Check sheet for the modelled part. Datum: model origin and axes. Units: mm. Face numbers are marked on the shaded views. A direction names the side the tool comes from. Coordinates: 2 decimals unless noted, no trailing zeros. Order: outer loops, then holes, each group sorted by start corner. A loop starts at its lowest first (then second) coordinate and runs counter-clockwise, first axis right, second up.
1. Cross-section at A-A (y = 81.5). Enter the section's corners in (x, z).
2. Gauge pin test, flat ends, axial feed: pin 1 Ø9 at (y, z) = (16.5, 39.5) entering from +X; pin 2 Ø5 at (x, z) = (-20.5, 28) entering from +Y; pin 3 Ø1 at (y, z) = (60.5, 18) entering from +X; pin 4 Ø16 at (x, y) = (-20.5, 47) entering from -Z. Record the tip position at first contact, or that the pin passes through.
3. Set-up check for the marked faces 1, 2, 3 and 4: record each of +Z, -Z, +X, -X, +Y, -Y from which the full face is reachable in a straight line by a thin tool's end or side.
4. Draft check along X on the marked faces 5, 6 and 7. Enter one of: released by +X, released by -X, zero draft, split by the parting line, or undercut.
5. Cross-section at B-B (x = -16.5). Enter the section's corners in (y, z), then the cut area to 3 significant figures.
6. Cross-section at D-D (z = 4.5). Enter the section's corners in (x, y).
7. Cross-section at C-C (z = -5.5). Enter the section's corners in (x, y).
8. Thickness scan on line 1 (Y direction, x = -14, z = 0); line 2 (Z direction, x = -18.25, y = 85); line 3 (X direction, y = 22, z = -12.5). Record the ranges inside material, lowest first.
Autodesk Inventor part; units mm, degrees
ref_plane "РабПлоскость1" through (10, 0, -50) normal (1, 0, 0) x (0, 0, -1)
ref_plane "YZ Plane" through (0, 0, 0) normal (1, 0, 0) x (0, 1, 0)
ref_plane "XZ Plane" through (0, 0, 0) normal (0, 1, 0) x (-1, 0, 0)
sketch "Эскиз1" plane through (0, 0, 0) normal (0, 1, 0) x (-1, 0, 0)
  line L0 (30, 50) -> (30, -50)
  line L1 (30, -50) -> (-30, -50)
  line L2 (-30, -50) -> (-30, 50)
  line L3 (-30, 50) -> (30, 50)
  point P0 (0, 0)
  dimension "d2" = 100
  dimension "d3" = 60
  dimension "d4" = 100
extrude "Выдавливание1" add sketch "Эскиз1" along normal blind 40
sketch "Эскиз2" plane through (30, 0, 50) normal (1, 0, 0) x (0, 0, -1)
  line L0 (30, 0) -> (70, 0)
  line L1 (20, 20) -> (80, 20)
  line L2 (80, 20) -> (70, 0)
  line L3 (20, 20) -> (30, 0)
  point P0 (50, 0)
  dimension "d8" = 40
  dimension "d11" = 60
extrude "Выдавливание2" cut sketch "Эскиз2" along normal mid plane 160
sketch "Эскиз4" plane through (0, 40, 0) normal (0, 1, 0) x (1, 0, 0)
  line L0 (30, -30) -> (30, 30)
  line L1 (30, -50) -> (30, 50)
  arc A0 (22.5, 15) -> (-2.5, 15) centre (10, 15) ccw
  arc A1 (-2.5, -15) -> (22.5, -15) centre (10, -15) ccw
  line L2 (-2.5, 15) -> (-2.5, -15)
  line L3 (22.5, 15) -> (22.5, -15)
  point P0 (0, 0)
extrude "Выдавливание5" cut sketch "Эскиз4" against normal blind 20
sketch "Эскиз5" plane through (-30, 0, 50) normal (-1, 0, 0) x (0, 0, 1)
  line L0 (0, 40) -> (-100, 40)
  line L1 (-100, 40) -> (-85, 40)
  line L2 (-85, 40) -> (-15, 40)
  line L3 (-85, 40) -> (-85, 60)
  line L4 (-85, 60) -> (-75, 60)
  line L5 (-15, 40) -> (-15, 60)
  line L6 (-15, 60) -> (-25, 60)
  line L7 (-25, 60) -> (-25, 85)
  line L8 (-75, 60) -> (-75, 85)
  arc A0 (-25, 85) -> (-75, 85) centre (-50, 85) ccw
  line L9 (-75, 85) -> (-25, 85)
  circle A1 centre (-50, 85) radius 12.5
  point P0 (-50, 0)
  dimension "d50" = 70
  dimension "d51" = 20
  dimension "d52" = 10
  dimension "d53" = 20
  dimension "d54" = 10
  dimension "d55" = 25
  dimension "d56" = 25
  dimension "d59" = 25
extrude "Выдавливание6" add sketch "Эскиз5" against normal blind 20 contours L0 L3 L4 L8 L9 A1 L7 L6 L5 | L9 A1 A0
ref_plane "РабПлоскость1" through (10, 0, -50) normal (1, 0, 0) x (0, 0, -1)
sketch "Эскиз6" plane through (0, 40, 0) normal (0, 1, 0) x (1, 0, 0)
  arc A0 (-2.5, -15) -> (22.5, -15) centre (10, -15) ccw
  line L0 (10, -15) -> (10, -69.4027)
  line L1 (10, -69.4027) -> (54.89, -69.4027)
  line L2 (54.89, -69.4027) -> (54.89, -15)
  line L3 (10, -15) -> (10, 0)
  line L4 (10, 0) -> (54.89, 0)
  line L5 (54.89, 0) -> (54.89, -15)
  point P0 (0, 0)
  dimension "d65" = 12.5
extrude "Выдавливание7" cut sketch "Эскиз6" against normal blind 80
properties part number "Урок"
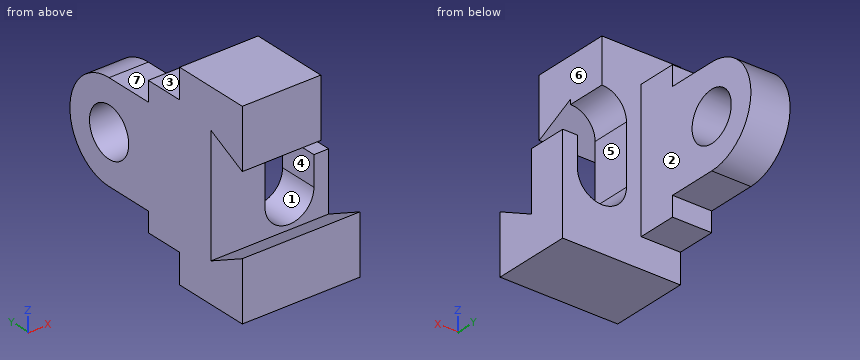
Data:
1. outline: (-30, -25) - (-10, -25) - (-10, -12) - (-30, -12) - close; (-30, 12) - (-10, 12) - (-10, 25) - (-30, 25) - close
2. pin 1: stops at x = 10
2. pin 2: stops at y = 60
2. pin 3: stops at x = -10
2. pin 4: stops at z = -50
3. face 1: +Y
3. face 2: +Z, -Z, +X, +Y
3. face 3: +Z, +X, -X, +Y
3. face 4: +Z, +Y, -Y
4. face 5: undercut
4. face 6: released by +X
4. face 7: zero draft
5. outline: (0, -50) - (40, -50) - (40, -35) - (60, -35) - (60, -25) - (85, -25) arc R25 ccw to (85, 25) - (60, 25) - (60, 35) - (40, 35) - (40, 50) - (0, 50) - (0, 20) - (20, 30) - (20, -30) - (0, -20) - close; hole circle Ø25 at (85, 0)
5. area: 6,140 mm2
6. outline: (-30, 20) - (-2.5, 20) - (-2.5, 40) - (-10, 40) - (-10, 73.34) - (-30, 73.34) - close; (-30, 96.66) - (-10, 96.66) - (-10, 109.59) - (-30, 109.59) - close
7. outline: (-30, 20) - (-2.5, 20) - (-2.5, 40) - (-10, 40) - (-10, 73.78) - (-30, 73.78) - close; (-30, 96.22) - (-10, 96.22) - (-10, 109.39) - (-30, 109.39) - close; (22.5, 20) - (30, 20) - (30, 40) - (22.5, 40) - close
8. line 1: y = 20 to 72.5, 97.5 to 110
8. line 2: z = -25 to -12.5, 12.5 to 25
8. line 3: x = -30 to -2.5, 22.5 to 30
